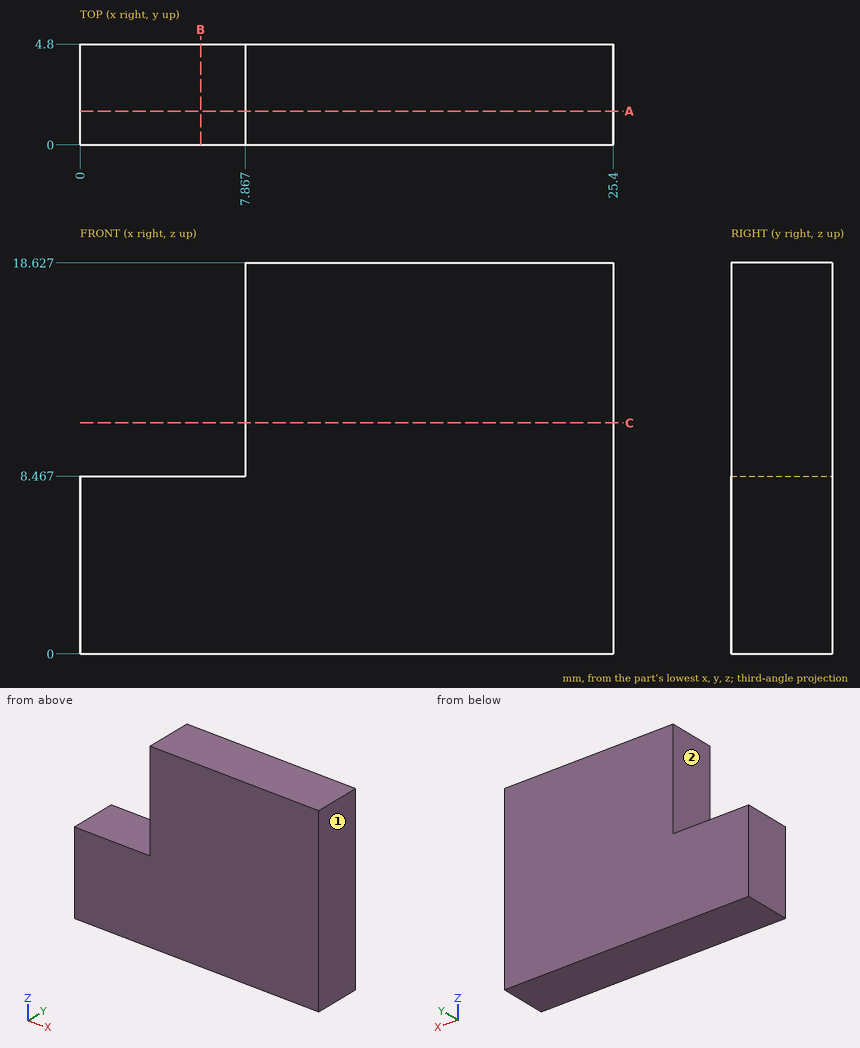
Geometry: see drawing. Coordinates: mm, zero at the bounding-box minimum. A direction names the side the tool comes from. Give positions to 0.01 mm unless a question says otherwise; leave off trailing zeros. Write each loop counter-clockwise with the first axis right and the second up, starting at its lowest first coordinate (ties: lowest second). Pieces come first, ordered by that corner, then holes. Notation, with made-up numbers: M 42,19.25 L 65,19.25 A27 ccw 65,56.25 Z; hole C 87.5,-31 d2. An arc over 180 degrees is marked long. Answer as a JSON object with one key per item and string values.
Q1. Cut plane B-B, the plane x = 5.75. Return the cut outline in (y, z).
Geometry check:
{"outline": "M 0,0 L 4.8,0 L 4.8,8.47 L 0,8.47 Z"}
Q2. Access query for the marked faces 1 and 2. Directions: +Z, -Z, +X, -X, +Y, -Y. A direction counts if a zero-diameter tool reaches every point of the face in a straight line with its end or side. Return the directions, or none.
Geometry check:
{"face 1": "+Z, -Z, +X, +Y, -Y", "face 2": "+Z, -X, +Y, -Y"}
Q3. Cut plane A-A, the plane y = 1.6. Return the cut outline in (x, z).
Geometry check:
{"outline": "M 0,0 L 25.4,0 L 25.4,18.63 L 7.87,18.63 L 7.87,8.47 L 0,8.47 Z"}
Q4. Contact query for flat-ended pins moving along their axis: P1, Ø1.4, axis at y = 2.5, z = 16, coming from the -X side; P2, Ø1, axis at x = 7.5, z = 14.5, coming from the -Y side; P3, Ø1.4, axis at x = 4.5, y = 3.5, coming from the +Z side. Output: stop coordinate, or through.
Geometry check:
{"P1": "stops at x = 7.87", "P2": "stops at y = 0", "P3": "stops at z = 8.47"}
Q5. Ray query, line 1 along X through (y, z) = (2.7, 17.25); line 2 along Z through (x, y) = (7.5, 3.85). Return the intervals inside material, ascending.
Geometry check:
{"line 1": "x = 7.87 to 25.4", "line 2": "z = 0 to 8.47"}
Q6. Cut plane C-C, the plane z = 11. Return the cut outline in (x, y).
Geometry check:
{"outline": "M 7.87,0 L 25.4,0 L 25.4,4.8 L 7.87,4.8 Z"}
